Source: three-view drawing plus pictorial views. Frame: mm from the lowest corner of the part. A direction names the side the tool comes from. Coordinates: 2 decimals unless noted, no trailing zeros. Loops run counter-clockwise (first coordinate to the right, second up) from the corner with the lowest first, then second, coordinate; pieces in that order, holes last. Notation, with made-up numbers: M 39.25,-36.75 L 84.25,-36.75 A15 ccw 84.25,-18.75 Z; hole C 38,62 d11. An arc over 180 degrees is marked long. Write each question's results on one line, items separated by ' | '. Start each with the question number.
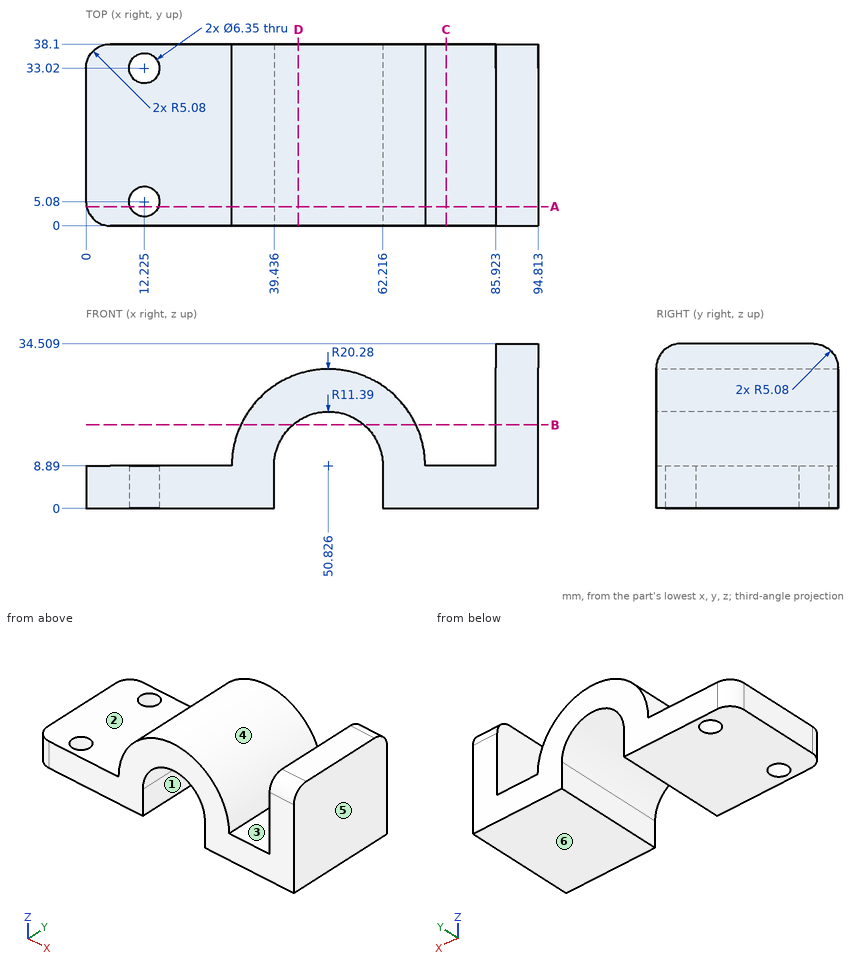
Item 1: Set-up query: the marked faces 1, 2 and 3. Return all of +Z, -Z, +X, -X, +Y, -Y with unobstructed straight access to the full face (end or side cutting, diameter ignored); none if empty.
Item 2: Section A-A, the plane y = 4. Return loops of the section in (x, z), plus the area to 3 significant figures.
Item 3: Section C-C, the plane x = 75.5. Return loops of the section in (y, z).
Item 4: Section B-B, the plane z = 17.5. Return loops of the section in (x, y), plus the area to 3 significant figures.
Item 5: Pull-direction query (X, two-part tool) for the marked faces 4, 5 and 6; classes: released by +X, released by -X, zero draft, split by the parting line, or undercut.
Item 6: Section D-D, the plane x = 44.5. Return loops of the section in (y, z).
Item 7: Ray query, L1, parallel to X at y = 5, z = 5; L2, parallel to X at y = 17, z = 9.5 (1 decimal); L3, parallel to Z at x = 29, y = 10.5. Return the intervals inside material, ascending. Write a range as [from, to].
Item 8: Contact query for flat-ended pins moving along their axis: P1, Ø9, axis at x = 18.5, y = 18.5, coming from the +Z side; P2, Ø12, axis at x = 23.5, z = 15.5, coming from the -Y side; P3, Ø1, axis at y = 8.5, z = 30, coming from the -X side; P4, Ø6, axis at x = 56.5, y = 13, coming from the -Z side. Output: stop coordinate, or through.
Solutions:
1) face 1: -Z, +Y, -Y | face 2: +Z, -X, +Y, -Y | face 3: +Z, +Y, -Y
2) outline: M 0.12,0 L 9.24,0 L 9.24,8.89 L 0.12,8.89 Z; M 15.21,0 L 39.44,0 L 39.44,8.89 A11.39 cw 62.22,8.89 L 62.22,0 L 94.81,0 L 94.81,34.39 L 85.92,34.39 L 85.92,8.89 L 71.11,8.89 A20.28 ccw 30.55,8.89 L 15.21,8.89 Z | area: 1,260 mm²
3) outline: M 0,0 L 38.1,0 L 38.1,8.89 L 0,8.89 Z
4) outline: M 32.46,0 L 43.37,0 L 43.37,38.1 L 32.46,38.1 Z; M 58.28,0 L 69.19,0 L 69.19,38.1 L 58.28,38.1 Z; M 85.92,0 L 94.81,0 L 94.81,38.1 L 85.92,38.1 Z | area: 1,170 mm²
5) face 4: undercut | face 5: released by +X | face 6: zero draft
6) outline: M 0,18.36 L 38.1,18.36 L 38.1,28.16 L 0,28.16 Z
7) L1: x = [0, 9.05], [15.4, 39.44], [62.22, 94.81] | L2: x = [30.6, 39.5], [62.2, 71.1], [85.9, 94.8] | L3: z = [0, 8.89]
8) P1: stops at z = 8.89 | P2: passes through | P3: stops at x = 85.92 | P4: stops at z = 16.27
